from build123d import *

# Parameters (mm, degrees)
SKETCH1_W           = 118.5
SKETCH1_H           = 92.5
SKETCH1_W_2         = 110.5
SKETCH1_H_2         = 84.5
BOSS_EXTRUDE1_DEPTH = 5
SKETCH2_R           = 2
SKETCH2_R_2         = 1.05
BOSS_EXTRUDE2_DEPTH = 5


with BuildPart() as part:
    # Sketch1 → Boss-Extrude1 (new body)
    with BuildSketch(Plane.XY):
        with Locations((59.25, 46.25)):
            Rectangle(SKETCH1_W, SKETCH1_H)
        with Locations((59.25, 46.25)):
            Rectangle(SKETCH1_W_2, SKETCH1_H_2, mode=Mode.SUBTRACT)
    extrude(amount=-BOSS_EXTRUDE1_DEPTH)

    # Sketch2 → Boss-Extrude2 (add)
    # profile 1 of 4: a face of its own
    with BuildSketch(Plane.XY):
        with Locations(Location((2, 90.5, 0), (0, 0, 180))):
            Circle(SKETCH2_R)
        with Locations((2, 90.5)):
            Circle(SKETCH2_R_2, mode=Mode.SUBTRACT)
    # profile 2 of 4: a face of its own
    with BuildSketch(Plane.XY):
        with Locations((116.5, 90.5)):
            Circle(SKETCH2_R)
        with Locations((116.5, 90.5)):
            Circle(SKETCH2_R_2, mode=Mode.SUBTRACT)
    # profile 3 of 4: a face of its own
    with BuildSketch(Plane.XY):
        with Locations((116.5, 2)):
            Circle(SKETCH2_R)
        with Locations((116.5, 2)):
            Circle(SKETCH2_R_2, mode=Mode.SUBTRACT)
    # profile 4 of 4: a face of its own
    with BuildSketch(Plane.XY):
        with Locations(Location((2, 2, 0), (0, 0, 180))):
            Circle(SKETCH2_R)
        with Locations((2, 2)):
            Circle(SKETCH2_R_2, mode=Mode.SUBTRACT)
    extrude(amount=BOSS_EXTRUDE2_DEPTH)


solid = part.part
Here's how the part is built. I have some questions about the finished solid (model axes, mm). A direction names the side the tool comes from. Give positions to 0.01 mm unless a question says otherwise; leave off trailing zeros. Order: outer loops, then holes, each group sorted by start corner. A loop starts at its lowest first (then second) coordinate and runs counter-clockwise, first axis right, second up. Notation, with made-up numbers: (10.25, 37) -> (15.25, 37) arc R10 ccw to (15.25, 43) -> close; hole circle Ø6 at (75, -11.5). An arc over 180 degrees is marked (long way). One line per item, written item: value. Start each with the question number.
1. We'd pull the mould along X, two halves only. Please class faces 1 (the face through (3.6, 3.2, 2.5)), 2 (the face through (118.5, 46, -2)), 3 (the face through (117.4, 89.6, 5)): released by +X, released by -X, zero draft, split by the parting line, or undercut.
2. For faces 4 (the face through (2.26, 88.517, 2.465)), 5 (the face through (58, 88.5, -2)), 6 (the face through (1.1, 91.4, 5)), which set-ups out of +Z, -Z, +X, -X, +Y, -Y let a thin tool reach every point of the face, with its end or its side?
3. Imagine slicing it at C-C, the plane z = -1.25. List the corners of the cut face in (x, y) for me.
4. Imagine slicing it at B-B, the plane x = 9. List the corners of the cut face in (y, z) for me, plus the area to 3 significant figures.
5. Will this pin go through, and if not, where does the flat tip stop? pin 1 Ø1.7 at (x, y) = (2, 2) entering from +Z.
6. Imagine slicing it at A-A, the plane y = 12.5. List the corners of the cut face in (x, z) for me, plus the area to 3 significant figures.
7. I need wall thicknesses on probe 1 along Y at (x, z) = (2, 1.75); probe 2 along X at (y, z) = (90.5, 2.9); probe 3 along X at (y, z) = (54, -3). Which ranges of each line are inside material? Lowest first, please. Write a range as from..to.
Values follow:
1. face 1: undercut
1. face 2: released by +X
1. face 3: zero draft
2. face 4: +Z
2. face 5: +Z, -Z
2. face 6: +Z, +X, -X, +Y, -Y
3. outline: (0, 0) -> (118.5, 0) -> (118.5, 92.5) -> (0, 92.5) -> close; hole (4, 4) -> (114.5, 4) -> (114.5, 88.5) -> (4, 88.5) -> close
4. outline: (0, -5) -> (4, -5) -> (4, 0) -> (0, 0) -> close; (88.5, -5) -> (92.5, -5) -> (92.5, 0) -> (88.5, 0) -> close
4. area: 40.0 mm2
5. pin 1: stops at z = 0
6. outline: (0, -5) -> (4, -5) -> (4, 0) -> (0, 0) -> close; (114.5, -5) -> (118.5, -5) -> (118.5, 0) -> (114.5, 0) -> close
6. area: 40.0 mm2
7. probe 1: y = 0..0.95, 3.05..4, 88.5..89.45, 91.55..92.5
7. probe 2: x = 0..0.95, 3.05..4, 114.5..115.45, 117.55..118.5
7. probe 3: x = 0..4, 114.5..118.5
